from build123d import *

# Parameters (mm, degrees)
ESQUISSE1_W        = 66.04
ESQUISSE1_H        = 53.34
ESQUISSE1_R        = 1.65
BOSS_EXTRU_1_DEPTH = 2
CONG_1_R           = 5


with BuildPart() as part:
    # Esquisse1 → Boss.-Extru.1 (new body)
    with BuildSketch(Plane(origin=(0, 0, 0), x_dir=(1, 0, 0), z_dir=(0, 1, 0))):
        Rectangle(ESQUISSE1_W, ESQUISSE1_H)
        with Locations((-27.94, 20.59)):
            Circle(ESQUISSE1_R, mode=Mode.SUBTRACT)
        with Locations((27.94, 20.59)):
            Circle(ESQUISSE1_R, mode=Mode.SUBTRACT)
        with Locations((27.94, -20.59)):
            Circle(ESQUISSE1_R, mode=Mode.SUBTRACT)
        with Locations((-27.94, -20.59)):
            Circle(ESQUISSE1_R, mode=Mode.SUBTRACT)
    extrude(amount=BOSS_EXTRU_1_DEPTH)

    # Congé1
    cong_1_edges = [part.edges().sort_by_distance(p)[0] for p in [
        (33.02, 1, 26.67),
        (-33.02, 1, 26.67),
        (-33.02, 1, -26.67),
        (33.02, 1, -26.67),
    ]]
    fillet(cong_1_edges, radius=CONG_1_R)


solid = part.part
Input: part model. Units: mm. Frame: model coordinates. Give positions to 0.01 mm unless a question says otherwise; leave off trailing zeros. Write each loop counter-clockwise with the first axis right and the second up, starting at its lowest first coordinate (ties: lowest second). Pieces come first, ordered by that corner, then holes.
Q1. Section B-B, the plane z = -20.59. Output: boundary loops of the cut face in (x, y).
Q2. Section A-A, the plane y = 0.95. Output: boundary loops of the cut face in (x, z).
Q3. Material intervals for probe 1 along Z at (x, y) = (-27.94, 1.2); probe 2 along X at (y, z) = (1, 20.59), sorted ascending.
Q4. Pull-direction query (X, two-part tool) for faces 1 (the face through (-31.59, 1.01, 25.17)), 2 (the face through (33.02, 1, 0)), 3 (the face through (26.63, 0.99, -19.59)), 4 (the face through (0, 1, -26.67)); classes: pulls with the +X half, pulls with the -X half, needs draft (parallel to the pull), parting line crosses it, or undercut.
Filled in:
1. outline: (-33.02, 0) - (-29.59, 0) - (-29.59, 2) - (-33.02, 2) - close; (-26.29, 0) - (26.29, 0) - (26.29, 2) - (-26.29, 2) - close; (29.59, 0) - (33.02, 0) - (33.02, 2) - (29.59, 2) - close
2. outline: (-33.02, -21.67) arc R5 ccw to (-28.02, -26.67) - (28.02, -26.67) arc R5 ccw to (33.02, -21.67) - (33.02, 21.67) arc R5 ccw to (28.02, 26.67) - (-28.02, 26.67) arc R5 ccw to (-33.02, 21.67) - close; hole circle Ø3.3 at (-27.94, -20.59); hole circle Ø3.3 at (-27.94, 20.59); hole circle Ø3.3 at (27.94, -20.59); hole circle Ø3.3 at (27.94, 20.59)
3. probe 1: z = -26.67 to -22.24, -18.94 to 18.94, 22.24 to 26.67
3. probe 2: x = -33.02 to -29.59, -26.29 to 26.29, 29.59 to 33.02
4. face 1: pulls with the -X half
4. face 2: pulls with the +X half
4. face 3: undercut
4. face 4: needs draft
